```python
from build123d import *

# Parameters (mm, degrees)
F0_R     = 85
F1_DEPTH = 129.6
F2_R     = 5
F3_DEPTH = 200
F4_R     = 40.25
F5_DEPTH = 1.5


with BuildPart() as f1:
    # F0 (on Top) → F1 (new body)
    with BuildSketch(Plane.XY):
        Circle(F0_R)
    extrude(amount=F1_DEPTH)

    # F2 (on Right) → F3 (join)
    with BuildSketch(Plane.YZ):
        with Locations((0, 42)):
            Circle(F2_R)
        with Locations((0, 111)):
            Circle(F2_R)
    extrude(amount=-F3_DEPTH)

    # F4 (on face) → F5 (cut)
    with BuildSketch(Plane(origin=(0, 0, 0), x_dir=(1, 0, 0), z_dir=(0, 0, -1))):
        Circle(F4_R)
    extrude(amount=-F5_DEPTH, mode=Mode.SUBTRACT)


solid = f1.part
```
Could you check a few things on this model? Use its own coordinates, in mm. A direction names the side the tool comes from. Round coordinates to 2 decimals unless told otherwise and drop trailing zeros. Loops run counter-clockwise (first coordinate to the right, second up) from the corner with the lowest first, then second, coordinate; pieces in that order, holes last. Notation, with made-up numbers: (23, -30.75) - (38, -30.75) arc R13 cw to (38, -8.75) - close; hole circle Ø1 at (50, 52.5). An arc over 180 degrees is marked (long way). Answer as CSV lines item,"result".
1. On a 3-axis mill with a long thin cutter (end or side, diameter ignored), from which of +Z, -Z, +X, -X, +Y, -Y can I reach the whole of each face in a straight line? I mean faces 1 (the face through (-200, 0, 42)), 2 (the face through (-1, -1, 1.5)), 3 (the face through (-141.62, -1.08, 106.12)). Say none if no direction works.
Filled in:
face 1,"+Z, -Z, -X, +Y, -Y"
face 2,"-Z"
face 3,"-X"
2. I want a section at A-A on y = 0. List the corners of the cut face in (x, z) for me.
Filled in:
outline,"(-200, 37) - (-85, 37) - (-85, 0) - (-40.25, 0) - (-40.25, 1.5) - (40.25, 1.5) - (40.25, 0) - (85, 0) - (85, 129.6) - (-85, 129.6) - (-85, 116) - (-200, 116) - (-200, 106) - (-85, 106) - (-85, 47) - (-200, 47) - close"
3. I want a section at D-D on x = -45. List the corners of the cut face in (y, z) for me, then the cut area to 3 significant figures.
Filled in:
outline,"(-72.11, 0) - (72.11, 0) - (72.11, 129.6) - (-72.11, 129.6) - close"
area,"18,700 mm^2"
4. Please list where these lines run through material, in increasing order: line 1 along Y through (x, z) = (0, 0.75); line 2 along Y through (x, z) = (-101.5, 38.5). Write a range as [from, to].
Filled in:
line 1,"y = [-85, -40.25], [40.25, 85]"
line 2,"y = [-3.57, 3.57]"
5. We'd pull the mould along X, two halves only. Please class faces 4 (the face through (-141.62, -0.651, 46.957)), 5 (the face through (-67.453, -51.721, 63.893)), 6 (the face through (-40.21, -1.77, 0.74)): +X half, -X half, draft (parallel to the pull), parting line (faces both ways), or undercut.
Filled in:
face 4,"draft"
face 5,"parting line"
face 6,"undercut"
6. I want a section at C-C on z = 103. List the corners of the cut face in (x, y) for me, then the cut area to 3 significant figures.
Filled in:
outline,"circle Ø170 at (0, 0)"
area,"22,700 mm^2"
7. For pin 1 Ø6 at (x, z) = (23.5, 71.5) entering from -Y; pin 2 Ø24 at (x, y) = (-8.5, 18) entering from -Z; pin 3 Ø2 at (x, z) = (44, 20.5) entering from +Y, each with a flat end and sliding along its axis, tell me the tip position at first contact or that it passes through.
Filled in:
pin 1,"stops at y = -82.49"
pin 2,"stops at z = 1.5"
pin 3,"stops at y = 73.32"
8. I want a section at B-B on x = -141. List the corners of the cut face in (y, z) for me, then the cut area to 3 significant figures.
Filled in:
outline,"circle Ø10 at (0, 42); circle Ø10 at (0, 111)"
area,"157 mm^2"
